Autodesk Inventor part; units mm, degrees
ref_plane "YZ Plane" through (0, 0, 0) normal (1, 0, 0) x (0, 1, 0)
ref_plane "XZ Plane" through (0, 0, 0) normal (0, 1, 0) x (-1, 0, 0)
ref_plane "XY Plane" through (0, 0, 0) normal (0, 0, 1) x (1, 0, 0)
sketch "Szkic1" plane through (0, 0, 0) normal (0, 0, 1) x (1, 0, 0)
  circle A0 centre (0, 0) radius 12.7
  dimension "d0" = 25.4
extrude "Wyciągnięcie proste1" add sketch "Szkic1" along normal blind 4.2 and the other way blind 5
sketch "Szkic2" plane through (0, 0, 0) normal (0, 0, 1) x (1, 0, 0)
  circle A0 centre (0, 0) radius 6
  circle A1 centre (0, 0) radius 12.7
  dimension "d5" = 12
extrude "Wyciągnięcie proste2" cut sketch "Szkic2" along normal blind 4.2
hole "Otwór1" at (0, 0, 4.2) direction (0, 0, -1) diameter 6 end through all
sketch "Szkic3" plane through (0, 0, 0) normal (0, 0, 1) x (1, 0, 0)
  line L0 (0, 0) -> (0, 9.5) construction
  dimension "d18" = 9.5
hole "Otwór2" at (0, 9.5, 0) direction (0, 0, -1) diameter 3 end through all
pattern_circular "Szyk kołowy1" count 6 over 360 about axis through (0, 0, -32.8805) along (0, 0, 1) of "Otwór2"
chamfer "Faza1" distance 0.25 angle 45 6 edges at (-6, 0, 4.2) (-12.7, 0, 0) (-12.7, 0, -5) (-6, 0, 0) (0, 3, -5) (0, 3, 4.2)
move or copy body "Przesuń bryłę1" bodies to move or copy 1 copy no rotation origin (0, 0, 0) rotation axis (0, 1, 0) rotation angle 180
properties part number "bepf_kolo_adapter_walu_fi6" material "Aluminium 6061"
The listing builds one solid part. Answer for the finished solid, in the listing's coordinates (mm). A direction names the side the tool comes from. Give positions to 0.01 mm unless a question says otherwise; leave off trailing zeros. Write each loop counter-clockwise with the first axis right and the second up, starting at its lowest first coordinate (ties: lowest second). Pieces come first, ordered by that corner, then holes.
1) Section B-B (y = 0) is taken. Write down the section's boundary in (x, z), and give its area (3 significant figures).
2) A tool of negligible diameter and unlimited length cuts with its end or side. For faces 1 (the face through (7.213, 3.644, 2.535)), 2 (the face through (-3, 6, 0)), from which of +Z, -Z, +X, -X, +Y, -Y can it reach the whole face along a straight path? Write none if from no direction.
3) For a pull along Y with two mould halves and no side action, classify faces 3 (the face through (2.75, -12.4, 2.47)), 4 (the face through (0, 3, 0)), 5 (the face through (-3, -3, 5)) as pulls with the +Y half, pulls with the -Y half, needs draft (parallel to the pull), parting line crosses it, or undercut.
4) Section A-A (x = 0) is taken. Count the separate pieces of the cut face and the enclosed holes in it, and give its area (4 significant figures).
5) Find the intervals of material crossed by L1, parallel to X at y = -4.75, z = 3.7; L2, parallel to Y at x = -7.5, z = 2.5; L3, parallel to Y at x = 0.25, z = 3.25, in increasing order.
6) Given P1, Ø3, axis at y = 2, z = -0.5, coming from the -X side; P2, Ø3, axis at x = 9, z = 4, coming from the +Y side; P3, Ø4, axis at x = -8.23, y = 4.75, coming from the -Z side; P4, Ø1.8, axis at x = 0, y = 9.5, coming from the -Z side, each flat-ended and moving along its own axis, determine where each tip first touches the part or whether it passes through.
7) Section C-C (z = -1.5) is taken. Write down the section's boundary in (x, y), and give its area (3 significant figures).
Response:
1. outline: (-12.7, 0.25) - (-12.45, 0) - (-6.25, 0) - (-6, -0.25) - (-6, -3.95) - (-5.75, -4.2) - (-3.25, -4.2) - (-3, -3.95) - (-3, 4.75) - (-3.25, 5) - (-12.45, 5) - (-12.7, 4.75) - close; (3, -3.95) - (3.25, -4.2) - (5.75, -4.2) - (6, -3.95) - (6, -0.25) - (6.25, 0) - (12.45, 0) - (12.7, 0.25) - (12.7, 4.75) - (12.45, 5) - (3.25, 5) - (3, 4.75) - close
1. area: 122 mm2
2. face 1: +Z, -Z
2. face 2: -Z
3. face 3: parting line crosses it
3. face 4: undercut
3. face 5: needs draft
4. separate pieces: 4
4. enclosed holes: 0
4. area: 91.95 mm2
5. L1: x = -11.78 to -9.73, -6.73 to 6.73, 9.73 to 11.78
5. L2: y = -10.25 to -6.06, -3.44 to 3.44, 6.06 to 10.25
5. L3: y = -12.7 to -10.98, -8.02 to -2.99, 2.99 to 8.02, 10.98 to 12.7
6. P1: stops at x = -12.68
6. P2: stops at y = 10.25
6. P3: stops at z = 0
6. P4: passes through
7. outline: circle Ø12 at (0, 0); hole circle Ø6 at (0, 0)
7. area: 84.8 mm2
